Build history of the part. All positions in model axes, mm. Coordinates: 2 decimals unless noted, no trailing zeros. Write each loop counter-clockwise with the first axis right and the second up, starting at its lowest first coordinate (ties: lowest second). Pieces come first, ordered by that corner, then holes.
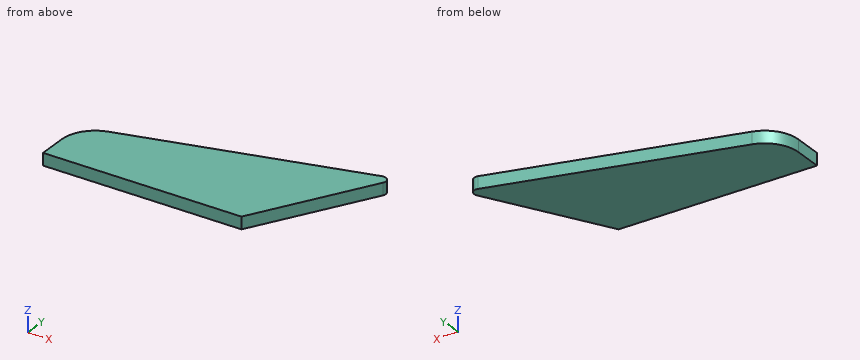
from build123d import *

# Parameters (mm, degrees)
BOSS_EXTRU_1_DEPTH = 18
CONG_1_R           = 50
CONG_2_R           = 9


with BuildPart() as part:
    # Esquisse1 → Boss.-Extru.1 (new body)
    with BuildSketch(Plane.XY):
        Polygon((0, 0), (295, 0), (403.62976321, 188.152269093), (0, 80), align=None)
    extrude(amount=BOSS_EXTRU_1_DEPTH)

    # Congé1
    cong_1_edges = [part.edges().sort_by_distance(p)[0] for p in [
        (0, 80, 9),
    ]]
    fillet(cong_1_edges, radius=CONG_1_R)

    # Congé2
    cong_2_edges = [part.edges().sort_by_distance(p)[0] for p in [
        (403.62976321, 188.152269093, 9),
    ]]
    fillet(cong_2_edges, radius=CONG_2_R)


solid = part.part
(1) Slice it at C-C, the plane x = 184. List the corners of the cut face in (y, z), and give its area (3 significant figures).
(2) Slice it at B-B, the plane y = 80.5. List the corners of the cut face in (x, z).
(3) Flat gauge pins, fed straight in: P1, Ø2, axis at y = 76.5, z = 2, coming from the -X side; P2, Ø4, axis at x = 217.5, z = 7, coming from the +Y side; P3, Ø2, axis at x = 48, z = 2.5, coming from the -Y side; P4, Ø3, axis at x = 139, z = 12.5, coming from the +Y side. Where does each tip first touch, or does it go through?
(4) Slice it at A-A, the plane z = 8. List the corners of the cut face in (x, y).
(5) Probe L1, parallel to Y at x = 329, z = 11.75; L2, parallel to Y at x = 314.5, z = 13 (3 decimals); L3, parallel to X at y = 42, z = 8.25. List the from-to ranges inside material, lowest first.
Results:
1. outline: (0, 0) - (129.3, 0) - (129.3, 18) - (0, 18) - close
1. area: 2,330 mm2
2. outline: (18.55, 0) - (341.48, 0) - (341.48, 18) - (18.55, 18) - close
3. P1: stops at x = 13.22
3. P2: stops at y = 138.81
3. P3: stops at y = 0
3. P4: stops at y = 117.65
4. outline: (0, 0) - (295, 0) - (392.77, 169.34) arc R9 ccw to (382.64, 182.53) - (37.06, 89.93) arc R50 ccw to (0, 41.63) - close
5. L1: y = 58.89 to 168.16
5. L2: y = 33.775 to 164.27
5. L3: x = 0 to 319.25
